Read the model definition and answer for the solid it produces. Units are mm, in the model's axes. A direction names the side the tool comes from. Coordinates: 2 decimals unless noted, no trailing zeros. Loops run counter-clockwise (first coordinate to the right, second up) from the corner with the lowest first, then second, coordinate; pieces in that order, holes last.
from build123d import *

# Parameters (mm, degrees)
BOSS_EXTRUDE1_DEPTH = 55
BOSS_EXTRUDE2_START = 2
BOSS_EXTRUDE2_DEPTH = 2
BOSS_EXTRUDE3_START = 2
BOSS_EXTRUDE3_DEPTH = 2
BOSS_EXTRUDE5_START = 2
BOSS_EXTRUDE5_DEPTH = 2
BOSS_EXTRUDE6_DEPTH = 2
SKETCH7_W           = 3.4
SKETCH7_H           = 11.3
CUT_EXTRUDE2_DEPTH  = 55
SKETCH8_R           = 2.15
CUT_EXTRUDE3_DEPTH  = 6
CUT_EXTRUDE4_REACH  = 111.395
SKETCH9_R           = 2.7
LPATTERN1_COUNT     = 2
LPATTERN1_PITCH     = 37
LPATTERN2_COUNT     = 2
LPATTERN2_PITCH     = 41


with BuildPart() as part:
    # Sketch1 → Boss-Extrude1 (new body)
    with BuildSketch(Plane.XY):
        with BuildLine():
            Line((0, 0), (0, -93.2))
            Line((0, -93.2), (-6, -93.2))
            Line((-6, -93.2), (-6, -81.2))
            Line((-6, -81.2), (-16, -81.2))
            Line((-16, -81.2), (-16, -74.2))
            ThreePointArc((-16, -74.2), (-8.4, -66.6), (-16, -59))
            Line((-16, -59), (-16, -44.3))
            Line((-16, -44.3), (-8.4, -44.3))
            Line((-8.4, -44.3), (-8.4, -37.6))
            Line((-8.4, -37.6), (-16, -37.6))
            Line((-16, -37.6), (-16, -34.2))
            ThreePointArc((-16, -34.2), (-8.4, -26.6), (-16, -19))
            Line((-16, -19), (-16, -12))
            Line((-16, -12), (-6, -12))
            Line((-6, -12), (-6, 0))
            Line((-6, 0), (0, 0))
        make_face()
    extrude(amount=BOSS_EXTRUDE1_DEPTH)

    # Sketch2 → Boss-Extrude2 (add)
    with BuildSketch(Plane(origin=(0, 0, 28.5), x_dir=(-1, 0, 0), z_dir=(0, 0, -1)).offset(BOSS_EXTRUDE2_START)):
        with BuildLine():
            Line((16, -34.2), (16, -31.5))
            ThreePointArc((16, -31.5), (11.1, -26.6), (16, -21.7))
            Line((16, -21.7), (16, -19))
            ThreePointArc((16, -19), (8.4, -26.6), (16, -34.2))
        make_face()
    extrude(amount=-BOSS_EXTRUDE2_DEPTH)

    # Sketch3 → Boss-Extrude3 (add)
    with BuildSketch(Plane(origin=(0, 0, 28.5), x_dir=(-1, 0, 0), z_dir=(0, 0, -1)).offset(BOSS_EXTRUDE3_START)):
        with BuildLine():
            Line((16, -74.2), (16, -71.5))
            ThreePointArc((16, -71.5), (11.1, -66.6), (16, -61.7))
            Line((16, -61.7), (16, -59))
            ThreePointArc((16, -59), (8.4, -66.6), (16, -74.2))
        make_face()
    extrude(amount=-BOSS_EXTRUDE3_DEPTH)

    # Sketch4 → Boss-Extrude5 (add)
    with BuildSketch(Plane(origin=(0, 0, 2), x_dir=(-1, 0, 0), z_dir=(0, 0, -1)).offset(BOSS_EXTRUDE5_START)):
        with BuildLine():
            Line((16, -59), (16, -61.7))
            ThreePointArc((16, -61.7), (11.1, -66.6), (16, -71.5))
            Line((16, -71.5), (16, -74.2))
            ThreePointArc((16, -74.2), (8.4, -66.6), (16, -59))
        make_face()
        with BuildLine():
            Line((16, -19), (16, -21.7))
            ThreePointArc((16, -21.7), (11.1, -26.6), (16, -31.5))
            Line((16, -31.5), (16, -34.2))
            ThreePointArc((16, -34.2), (8.4, -26.6), (16, -19))
        make_face()
    extrude(amount=-BOSS_EXTRUDE5_DEPTH)

    # Sketch5 → Boss-Extrude6 (add)
    with BuildSketch(Plane(origin=(0, 0, 53), x_dir=(-1, 0, 0), z_dir=(0, 0, -1))):
        with BuildLine():
            Line((16, -19), (16, -21.7))
            ThreePointArc((16, -21.7), (11.1, -26.6), (16, -31.5))
            Line((16, -31.5), (16, -34.2))
            ThreePointArc((16, -34.2), (8.4, -26.6), (16, -19))
        make_face()
        with BuildLine():
            Line((16, -59), (16, -61.7))
            ThreePointArc((16, -61.7), (11.1, -66.6), (16, -71.5))
            Line((16, -71.5), (16, -74.2))
            ThreePointArc((16, -74.2), (8.4, -66.6), (16, -59))
        make_face()
    extrude(amount=-BOSS_EXTRUDE6_DEPTH)

    # Sketch7 → Cut-Extrude2 (cut)
    with BuildSketch(Plane.XY.offset(55)):
        with Locations((-14.3, -49.95)):
            Rectangle(SKETCH7_W, SKETCH7_H)
    extrude(amount=-CUT_EXTRUDE2_DEPTH, mode=Mode.SUBTRACT)

    # Sketch8 → Cut-Extrude3 (cut)
    with BuildSketch(Plane(origin=(0, 0, 0), x_dir=(0, 0, -1), z_dir=(1, 0, 0))):
        with Locations(Location((-46, -6, 0), (0, 0, 90))):
            Circle(SKETCH8_R)
        with Locations(Location((-9, -6, 0), (0, 0, 90))):
            Circle(SKETCH8_R)
        with Locations(Location((-7, -87.2, 0), (0, 0, 90))):
            Circle(SKETCH8_R)
        with Locations(Location((-48, -87.2, 0), (0, 0, 90))):
            Circle(SKETCH8_R)
    extrude(amount=-CUT_EXTRUDE3_DEPTH, mode=Mode.SUBTRACT)

    # Cut-Extrude4: up to this face of the body (flat: up to its plane)
    cut_extrude4_end = Plane(part.part.faces().sort_by_distance((-12.6, -49.95, 27.5))[0])
    # Sketch9 → Cut-Extrude4 (cut, up to the picked face)
    with BuildSketch(Plane(origin=(0, 0, 0), x_dir=(0, 0, -1), z_dir=(1, 0, 0)), mode=Mode.PRIVATE) as cut_extrude4_sk1:
        with Locations(Location((-27.5, -46.6, 0), (0, 0, 90))):
            Circle(SKETCH9_R)
    cut_extrude4_tool1 = split(extrude(cut_extrude4_sk1.sketch, amount=-CUT_EXTRUDE4_REACH, mode=Mode.PRIVATE), bisect_by=cut_extrude4_end, keep=Keep.BOTH, mode=Mode.PRIVATE)
    add(cut_extrude4_tool1.solids().sort_by(Axis((0, -46.6, 27.5), (-1, 0, 0)))[0], mode=Mode.SUBTRACT)

    # Cut-Loft1: read off the stored shape, not the designer's step
    # Cut-Loft1: loft between two sections, ruled curve by curve
    cut_loft1_from = [
        Edge.make_bspline([(0, -9.090752309, 49.270665095), (0, -2.54942212, 55.452169714), (0, 3.632082499, 48.910839524), (0, -2.909247691, 42.729334905), (0, -9.45057788, 36.547830286), (0, -15.632082499, 43.089160476), (0, -9.090752309, 49.270665095)], [0, 0, 0, 0, 0.5, 0.5, 0.5, 1, 1, 1, 1], 3, [1, 0.333333333, 0.333333333, 1, 0.333333333, 0.333333333, 1]),
    ]
    cut_loft1_to = [
        Edge.make_bspline([(-2.5, -7.797727139, 47.179269746), (-2.5, -5.439187646, 50.774724024), (-2.5, -1.843733369, 48.416184531), (-2.5, -4.202272861, 44.820730254), (-2.5, -6.560812354, 41.225275976), (-2.5, -10.156266631, 43.583815469), (-2.5, -7.797727139, 47.179269746)], [0, 0, 0, 0, 0.5, 0.5, 0.5, 1, 1, 1, 1], 3, [1, 0.333333333, 0.333333333, 1, 0.333333333, 0.333333333, 1]),
    ]
    cut_loft1 = Solid(Shell([*[Face.make_surface_from_curves(cut_loft1_from[k], cut_loft1_to[k]) for k in range(1)], Face(Wire(cut_loft1_from)), Face(Wire(cut_loft1_to))]))
    add(cut_loft1, mode=Mode.SUBTRACT)

    # LPattern1: Cut-Loft1 ×2
    with Locations(*[(0, 0, -i * LPATTERN1_PITCH) for i in range(1, LPATTERN1_COUNT)]):
        add(cut_loft1, mode=Mode.SUBTRACT)

    # Cut-Loft2: read off the stored shape, not the designer's step
    # Cut-Loft2: loft between two sections, ruled curve by curve
    cut_loft2_from = [
        Edge.make_bspline([(-2.5, -88.803773463, 46.568074485), (-2.5, -85.939922433, 43.36052756), (-2.5, -82.732375507, 46.22437859), (-2.5, -85.596226537, 49.431925515), (-2.5, -88.460077567, 52.63947244), (-2.5, -91.667624493, 49.77562141), (-2.5, -88.803773463, 46.568074485)], [0, 0, 0, 0, 0.5, 0.5, 0.5, 1, 1, 1, 1], 3, [1, 0.333333333, 0.333333333, 1, 0.333333333, 0.333333333, 1]),
    ]
    cut_loft2_to = [
        Edge.make_bspline([(0, -88.245004687, 43.623018711), (0, -79.491042109, 41.533009337), (0, -77.401032735, 50.286971915), (0, -86.154995313, 52.376981289), (0, -94.908957891, 54.466990663), (0, -96.998967265, 45.713028085), (0, -88.245004687, 43.623018711)], [0, 0, 0, 0, 0.5, 0.5, 0.5, 1, 1, 1, 1], 3, [1, 0.333333333, 0.333333333, 1, 0.333333333, 0.333333333, 1]),
    ]
    cut_loft2 = Solid(Shell([*[Face.make_surface_from_curves(cut_loft2_from[k], cut_loft2_to[k]) for k in range(1)], Face(Wire(cut_loft2_from)), Face(Wire(cut_loft2_to))]))
    add(cut_loft2, mode=Mode.SUBTRACT)

    # LPattern2: Cut-Loft2 ×2
    with Locations(*[(0, 0, -i * LPATTERN2_PITCH) for i in range(1, LPATTERN2_COUNT)]):
        add(cut_loft2, mode=Mode.SUBTRACT)


solid = part.part
Q1. A cutting plane is placed at A-A (y = -46.6). Give the vertices of the cut face in (x, z).
Findings below:
outline: (-12.6, 0) - (0, 0) - (0, 24.8) - (-12.6, 24.8) - close; (-12.6, 30.2) - (0, 30.2) - (0, 55) - (-12.6, 55) - close
Q2. Which of the six approach directions +Z, -Z, +X, -X, +Y, -Y give full straight-line access (tool end or side, diameter ignored) to faces 1 (the face through (-8.4, -26.77, 40.58)), 2 (the face through (-12, -37.6, 27)), 3 (the face through (-6, -6, 27))?
Findings below:
face 1: -X
face 2: +Z, -Z, -X
face 3: +Z, -Z, -X, +Y
Q3. Determine the mould class of faces 4 (the face through (-4.23, -87.67, 45.9)), 5 (the face through (0, -46, 33)), 6 (the face through (-11, -81.2, 27)) for opening direction Y: +Y half, -Y half, draft (parallel to the pull), parting line (faces both ways), or undercut.
Findings below:
face 4: undercut
face 5: draft
face 6: -Y half
Q4. A cutting plane is placed at D-D (y = -6). Count the separate pieces of the cut face and the enclosed holes in it, then the cut area to 3 significant figures.
Findings below:
separate pieces: 3
enclosed holes: 0
area: 267 mm2
Q5. A cutting plane is placed at B-B (z = 27.5). Give the vertices of the cut face in (x, y), then the cut area to 3 significant figures.
Findings below:
outline: (-16, -81.2) - (-6, -81.2) - (-6, -93.2) - (0, -93.2) - (0, -49.3) - (-12.6, -49.3) - (-12.6, -55.6) - (-16, -55.6) - (-16, -61.7) arc R4.9 cw to (-16, -71.5) - close; (-16, -37.6) - (-8.4, -37.6) - (-8.4, -43.9) - (0, -43.9) - (0, 0) - (-6, 0) - (-6, -12) - (-16, -12) - (-16, -21.7) arc R4.9 cw to (-16, -31.5) - close
area: 1,020 mm2
Q6. Straight lines are drawn through the part: probe 1 along Z at (x, y) = (-5.05, -87.2); probe 2 along Y at (x, z) = (-10, 27.5); probe 3 along X at (y, z) = (-5, 36). For each, find the intervals that lie inside material, in ascending order.
Findings below:
probe 1: z = 0 to 4.85, 9.15 to 45.85, 50.15 to 55
probe 2: y = -81.2 to -49.3, -37.6 to -12
probe 3: x = -6 to 0
Q7. Flat-ended cylindrical pins translate along their axes: pin 1 Ø2 at (x, z) = (-10.5, 42) entering from +Y; pin 2 Ø3.5 at (y, z) = (-8.5, 17) entering from -X; pin 3 Ø5 at (y, z) = (-87.2, 7) entering from +X. Find the tip coordinate at first contact, or state that the pin passes through.
Findings below:
pin 1: stops at y = -12
pin 2: stops at x = -6
pin 3: stops at x = -2.01
Q8. A cutting plane is placed at C-C (y = -66.6). Give the vertices of the cut face in (x, z).
Findings below:
outline: (-11.1, 0) - (0, 0) - (0, 55) - (-11.1, 55) - (-11.1, 53) - (-8.4, 53) - (-8.4, 28.5) - (-11.1, 28.5) - (-11.1, 26.5) - (-8.4, 26.5) - (-8.4, 2) - (-11.1, 2) - close
